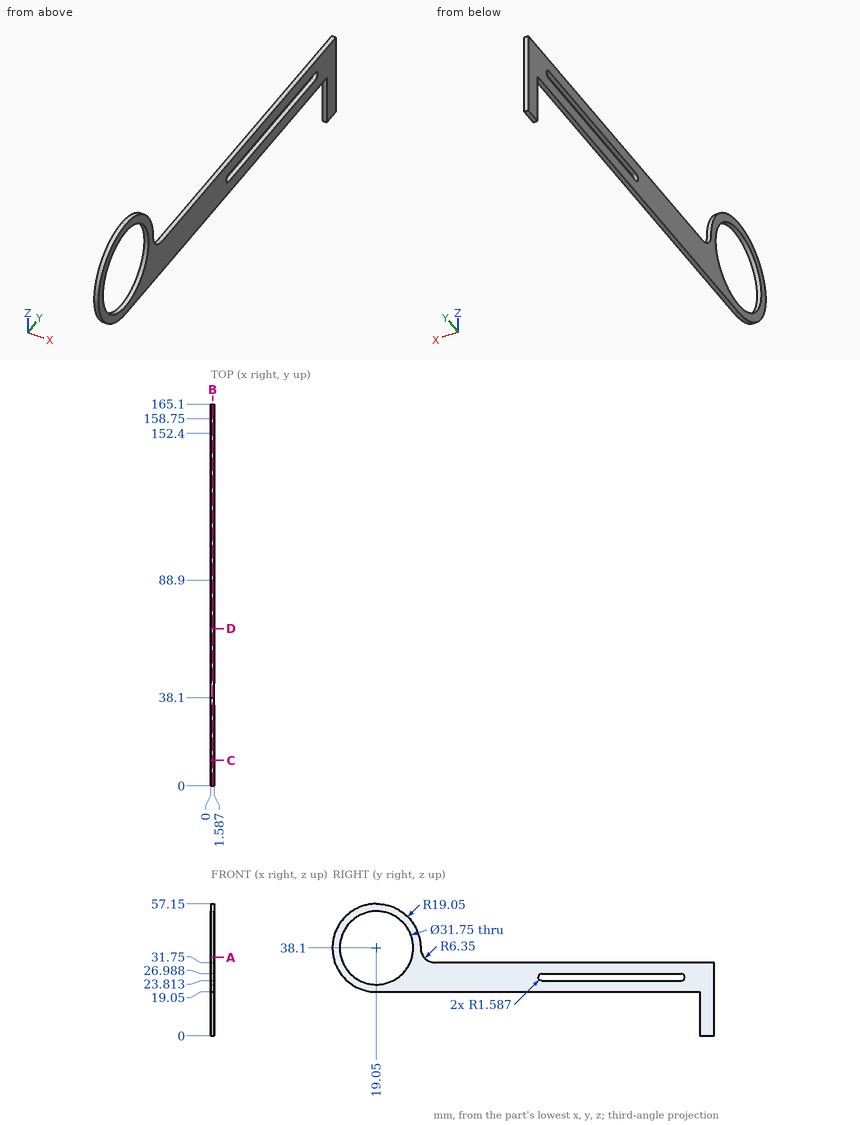
Study the drawing (mm; zero at the part's minimum x, y, z) and answer. Round coordinates to 2 decimals unless told otherwise and drop trailing zeros. Write each loop counter-clockwise with the first axis right and the second up, starting at its lowest first coordinate (ties: lowest second). Pieces come first, ordered by that corner, then holes.
1) A cutting plane is placed at A-A on z = 34. Determine the outline of the cut face in (x, y).
2) A cutting plane is placed at C-C on y = 11. Determine the outline of the cut face in (x, z) (1 decimal), and give its area (3 significant figures).
3) A cutting plane is placed at D-D on y = 68. Determine the outline of the cut face in (x, z).
4) Consider probe 1 along Z at (x, y) = (1.15, 110); probe 2 along Y at (x, z) = (0.3, 39); probe 3 along Z at (x, y) = (1.5, 47). Determine where each line is inside the solid, lowest interval first.
5) Flat-ended cylindrical pins translate along their axes: P1, Ø0.5, axis at x = 1, y = 116.5, coming from the -Z side; P2, Ø0.8, axis at x = 1, y = 95, coming from the +Z side; P3, Ø0.5, axis at x = 0.5, z = 10.5, coming from the -Y side. Find the tip coordinate at first contact, or state that the pin passes through.
6) A cutting plane is placed at B-B on x = 0.85. Give the number of separate pieces and of enclosed holes in the cut face, and give its area (3 significant figures).
Entries:
1. outline: (0, 0.45) - (1.59, 0.45) - (1.59, 3.71) - (0, 3.71) - close; (0, 34.39) - (1.59, 34.39) - (1.59, 39.6) - (0, 39.6) - close
2. outline: (0, 20.8) - (1.6, 20.8) - (1.6, 24.4) - (0, 24.4) - close; (0, 51.8) - (1.6, 51.8) - (1.6, 55.4) - (0, 55.4) - close
2. area: 11.4 mm2
3. outline: (0, 19.05) - (1.59, 19.05) - (1.59, 31.75) - (0, 31.75) - close
4. probe 1: z = 19.05 to 23.81, 26.99 to 31.75
4. probe 2: y = 0.02 to 3.2, 34.9 to 38.08
4. probe 3: z = 19.05 to 31.75
5. P1: stops at z = 19.05
5. P2: stops at z = 31.75
5. P3: stops at y = 158.75
6. separate pieces: 1
6. enclosed holes: 2
6. area: 1,970 mm2
